Geometry check sheet. Reference: the model listing, model coordinates, mm. Give positions to 0.01 mm unless a question says otherwise; leave off trailing zeros. Loops run counter-clockwise (first coordinate to the right, second up) from the corner with the lowest first, then second, coordinate; pieces in that order, holes last. Notation, with made-up numbers: (51.5, -18) -> (86.5, -18) arc R22 ccw to (86.5, -9) -> close; hole circle Ø7 at (3, 31). An arc over 180 degrees is marked (long way). One line per item, written item: value. Start each with the question number.
(1) Draft check along Z on faces 1 (the face through (0.84, 0.21, 21.43)), 2 (the face through (62.545, 8.62, -0.167)), 3 (the face through (0.84, 0.21, -21.43)). Enter one of: pulls with the +Z half, pulls with the -Z half, needs draft (parallel to the pull), parting line crosses it, or undercut.
(2) Gauge pin test, flat ends, axial feed: pin 1 Ø1 at (x, y) = (25.5, 4.5) entering from +Z; pin 2 Ø6 at (x, y) = (33.5, 6.5) entering from -Z; pin 3 Ø1 at (x, y) = (-19.5, -1) entering from +Z. Record the tip position at first contact, or that the pin passes through.
(3) Scan lines: line 1 along Z through (x, y) = (40, -0.25); line 2 along Z through (x, y) = (7, -7.5); line 3 along Y through (x, z) = (25, 16.5). Record each from-to range of solid material in increasing order. Write a range as from..to.
(4) Sectioned sample at A-A, the plane x = -52.5. Record the cut outline in (y, z) (3 decimals), then the cut area to 3 significant figures.
from build123d import *

# Parameters (mm, degrees)
SKETCH1_W           = 23.8125
SKETCH1_H           = 19.05
BOSS_EXTRUDE1_DEPTH = 63.5
FILLET1_R           = 3.175


with BuildPart() as part:
    # Sketch1 → Boss-Extrude1 (new body, symmetric)
    with BuildSketch(Plane(origin=(0, 0, 0), x_dir=(0, 0, -1), z_dir=(1, 0, 0))):
        with BuildLine():
            Line((-11.90625, -9.525), (-11.90625, 9.525))
            ThreePointArc((-11.90625, 9.525), (-21.43125, 0), (-11.90625, -9.525))
        make_face()
        Rectangle(SKETCH1_W, SKETCH1_H)
        with BuildLine():
            ThreePointArc((11.90625, 9.525), (21.43125, 0), (11.90625, -9.525))
            Line((11.90625, -9.525), (11.90625, 9.525))
        make_face()
    extrude(amount=BOSS_EXTRUDE1_DEPTH, both=True)

    # Fillet1
    fillet1_edges = [part.edges().sort_by_distance(p)[0] for p in [
        (63.5, 0, -21.43125),
        (63.5, 9.525, 0),
        (63.5, 0, 21.43125),
        (-63.5, 9.525, 0),
        (-63.5, 0, -21.43125),
        (-63.5, -9.525, 0),
        (-63.5, 0, 21.43125),
        (63.5, -9.525, 0),
    ]]
    fillet(fillet1_edges, radius=FILLET1_R)


solid = part.part
Calculated:
1. face 1: pulls with the +Z half
1. face 2: needs draft
1. face 3: pulls with the -Z half
2. pin 1: stops at z = 20.55
2. pin 2: stops at z = -20.76
2. pin 3: stops at z = 21.42
3. line 1: z = -21.43..21.43
3. line 2: z = -17.78..17.78
3. line 3: y = -8.34..8.34
4. outline: (-9.525, -11.906) arc R9.525 ccw to (9.525, -11.906) -> (9.525, 11.906) arc R9.525 ccw to (-9.525, 11.906) -> close
4. area: 739 mm2
